from build123d import *

# Parameters (mm, degrees)
BOSS_EXTRUDE1_DEPTH      = 20.32
SKETCH2_W                = 58.42
SKETCH2_H                = 52.07
BOSS_EXTRUDE2_DEPTH      = 3.81
SKETCH3_W                = 12.7
SKETCH3_H                = 20.32
CUT_EXTRUDE1_DEPTH       = 3.81
FILLET2_R                = 2.54
SKETCH4_W                = 10.16
SKETCH4_H                = 5.08
BOSS_EXTRUDE3_DEPTH      = 10.16
CHAMFER1_SIZE            = 0.762
SKETCH5_W                = 10.16
SKETCH5_H                = 5.08
BOSS_EXTRUDE4_DEPTH      = 10.16
CHAMFER2_SIZE            = 0.762
CHAMFER2_OF_MIRROR1_SIZE = 0.762
M3_CLEARANCE_HOLE1_D     = 3.4
M3_CLEARANCE_HOLE2_D     = 3.4
CUT_EXTRUDE2_REACH       = 61.966
SKETCH13_W               = 44.45
SKETCH13_H               = 16.51
SKETCH15_W               = 13.462
SKETCH15_H               = 7.366
CUT_EXTRUDE4_DEPTH       = 79.475827011
FILLET3_R                = 2.54
SKETCH16_W               = 6.35
SKETCH16_H               = 3.81
BOSS_EXTRUDE5_DEPTH      = 3.81
CHAMFER3_SIZE            = 0.762
M3_CLEARANCE_HOLE4_D     = 3.4
CUT_EXTRUDE5_DEPTH       = 3.302


with BuildPart() as part:
    # Sketch1 → Boss-Extrude1 (new body)
    with BuildSketch(Plane(origin=(0, 0, 0), x_dir=(1, 0, 0), z_dir=(0, 1, 0))):
        Polygon((-27.305, 22.225), (-27.305, 26.035), (31.115, 26.035), (31.115, -26.035), (-27.305, -26.035), (-27.305, -22.225), (27.305, -22.225), (27.305, 22.225), align=None)
    extrude(amount=BOSS_EXTRUDE1_DEPTH)

    # Sketch2 → Boss-Extrude2 (add)
    with BuildSketch(Plane(origin=(0, 20.32, 0), x_dir=(1, 0, 0), z_dir=(0, 1, 0))):
        with Locations((1.905, 0)):
            Rectangle(SKETCH2_W, SKETCH2_H)
    extrude(amount=BOSS_EXTRUDE2_DEPTH)

    # Sketch3 → Cut-Extrude1 (cut)
    with BuildSketch(Plane.ZY.offset(-27.305)):
        with Locations((-15.875, 10.16)):
            Rectangle(SKETCH3_W, SKETCH3_H)
        with Locations((15.875, 10.16)):
            Rectangle(SKETCH3_W, SKETCH3_H)
    extrude(amount=-CUT_EXTRUDE1_DEPTH, mode=Mode.SUBTRACT)

    # Fillet2
    fillet2_edges = [part.edges().sort_by_distance(p)[0] for p in [
        (31.115, 12.065, -26.035),
        (31.115, 12.065, 26.035),
        (31.115, 24.13, 0),
    ]]
    fillet(fillet2_edges, radius=FILLET2_R)

    # Sketch4 → Boss-Extrude3 (add)
    with BuildSketch(Plane(origin=(31.115, 0, 0), x_dir=(0, 0, -1), z_dir=(1, 0, 0))):
        with Locations((0, 2.54)):
            Rectangle(SKETCH4_W, SKETCH4_H)
    extrude(amount=BOSS_EXTRUDE3_DEPTH)

    # Chamfer1
    chamfer1_edges = [part.edges().sort_by_distance(p)[0] for p in [
        (31.115, 2.54, 5.08),
        (36.195, 5.08, 5.08),
        (31.115, 2.54, -5.08),
        (31.115, 5.08, 0),
        (36.195, 5.08, -5.08),
        (41.275, 2.54, 5.08),
        (41.275, 2.54, -5.08),
        (41.275, 5.08, 0),
    ]]
    chamfer(chamfer1_edges, length=CHAMFER1_SIZE)

    # Sketch5 → Boss-Extrude4 (add)
    with BuildSketch(Plane.XY.offset(26.035)):
        with Locations((-14.605, 2.54)):
            Rectangle(SKETCH5_W, SKETCH5_H)
    boss_extrude4 = extrude(amount=BOSS_EXTRUDE4_DEPTH)

    # Chamfer2
    chamfer2_edges = [part.edges().sort_by_distance(p)[0] for p in [
        (-19.685, 2.54, 26.035),
        (-19.685, 5.08, 31.115),
        (-9.525, 2.54, 26.035),
        (-14.605, 5.08, 26.035),
        (-9.525, 5.08, 31.115),
        (-19.685, 2.54, 36.195),
        (-9.525, 2.54, 36.195),
        (-14.605, 5.08, 36.195),
    ]]
    chamfer(chamfer2_edges, length=CHAMFER2_SIZE)

    # Mirror1: Boss-Extrude4 across plane
    add(boss_extrude4.mirror(Plane.XY))

    # Chamfer2 of Mirror1
    chamfer2_of_mirror1_edges = [part.edges().sort_by_distance(p)[0] for p in [
        (-19.685, 2.54, -26.035),
        (-19.685, 5.08, -31.115),
        (-9.525, 2.54, -26.035),
        (-14.605, 5.08, -26.035),
        (-9.525, 5.08, -31.115),
        (-19.685, 2.54, -36.195),
        (-9.525, 2.54, -36.195),
        (-14.605, 5.08, -36.195),
    ]]
    chamfer(chamfer2_of_mirror1_edges, length=CHAMFER2_OF_MIRROR1_SIZE)

    # M3 Clearance Hole1 (through all)
    with Locations(Plane(origin=(0, 5.08, 0), x_dir=(1, 0, 0), z_dir=(0, 1, 0))):
        with Locations((-14.605, -31.115)):
            m3_clearance_hole1 = Hole(M3_CLEARANCE_HOLE1_D / 2)

    # Mirror2: M3 Clearance Hole1 across plane
    add(m3_clearance_hole1.mirror(Plane.XY), mode=Mode.SUBTRACT)

    # M3 Clearance Hole2 (through all)
    with Locations(Plane(origin=(0, 5.08, 0), x_dir=(1, 0, 0), z_dir=(0, 1, 0))):
        with Locations((36.195, 0)):
            Hole(M3_CLEARANCE_HOLE2_D / 2)

    # Sketch13 → Cut-Extrude2 (cut, up to next)
    with BuildSketch(Plane(origin=(0, 24.13, 0), x_dir=(1, 0, 0), z_dir=(0, 1, 0)), mode=Mode.PRIVATE) as cut_extrude2_sk1:
        with Locations((0, -10.795)):
            Rectangle(SKETCH13_W, SKETCH13_H)
    cut_extrude2_tool1 = extrude(cut_extrude2_sk1.sketch, amount=-CUT_EXTRUDE2_REACH, mode=Mode.PRIVATE) & part.part
    # Sketch13 → Cut-Extrude2 (cut, up to next)
    with BuildSketch(Plane(origin=(0, 24.13, 0), x_dir=(1, 0, 0), z_dir=(0, 1, 0)), mode=Mode.PRIVATE) as cut_extrude2_sk2:
        with Locations((0, 10.795)):
            Rectangle(SKETCH13_W, SKETCH13_H)
    cut_extrude2_tool2 = extrude(cut_extrude2_sk2.sketch, amount=-CUT_EXTRUDE2_REACH, mode=Mode.PRIVATE) & part.part
    add(cut_extrude2_tool1.solids().sort_by_distance((0, 24.13, 10.795))[0], mode=Mode.SUBTRACT)
    add(cut_extrude2_tool2.solids().sort_by_distance((0, 24.13, -10.795))[0], mode=Mode.SUBTRACT)

    # Sketch15 → Cut-Extrude4 (cut, through all)
    with BuildSketch(Plane(origin=(0, 0, -26.035), x_dir=(-1, 0, 0), z_dir=(0, 0, -1))):
        Polygon((-22.225, 0), (4.953, 0), (4.953, 9.652), (4.953, 17.018), (2.441043817, 17.018), (-22.225, 17.018), align=None)
        with Locations((15.494, 13.335)):
            Rectangle(SKETCH15_W, SKETCH15_H)
    extrude(amount=-CUT_EXTRUDE4_DEPTH, mode=Mode.SUBTRACT)

    # Fillet3
    fillet3_edges = [part.edges().sort_by_distance(p)[0] for p in [
        (-22.225, 22.225, 19.05),
        (-22.225, 22.225, 2.54),
        (1.905, 20.32, -22.225),
        (22.225, 22.225, 2.54),
        (22.225, 22.225, 19.05),
        (22.225, 22.225, -19.05),
        (22.225, 22.225, -2.54),
        (-22.225, 22.225, -2.54),
        (-22.225, 22.225, -19.05),
        (22.225, 17.018, 24.13),
        (22.225, 17.018, -24.13),
        (-4.953, 17.018, 24.13),
        (-4.953, 17.018, -24.13),
        (-22.225, 17.018, 24.13),
        (-22.225, 17.018, -24.13),
        (-22.225, 9.652, 24.13),
        (-22.225, 9.652, -24.13),
        (-8.763, 9.652, 24.13),
        (-8.763, 9.652, -24.13),
        (-8.763, 17.018, 24.13),
        (-8.763, 17.018, -24.13),
        (29.21, 20.32, -9.525),
        (29.21, 20.32, 9.525),
        (1.905, 20.32, 22.225),
    ]]
    fillet(fillet3_edges, radius=FILLET3_R)

    # Sketch16 → Boss-Extrude5 (add)
    with BuildSketch(Plane(origin=(0, 24.13, 0), x_dir=(1, 0, 0), z_dir=(0, 1, 0))):
        with Locations((-27.305, 0)):
            Rectangle(SKETCH16_W, SKETCH16_H)
    extrude(amount=-BOSS_EXTRUDE5_DEPTH)

    # Chamfer3
    chamfer3_edges = [part.edges().sort_by_distance(p)[0] for p in [
        (-28.8925, 20.32, -1.905),
        (-28.8925, 20.32, 1.905),
        (-30.48, 20.32, 0),
        (-30.48, 22.225, -1.905),
        (-30.48, 22.225, 1.905),
    ]]
    chamfer(chamfer3_edges, length=CHAMFER3_SIZE)

    # M3 Clearance Hole4 (through all)
    with Locations(Plane(origin=(0, 24.13, 0), x_dir=(1, 0, 0), z_dir=(0, 1, 0))):
        with Locations((25.286866606, -21.9964), (25.286866606, 21.9964)):
            Hole(M3_CLEARANCE_HOLE4_D / 2)

    # Sketch22 → Cut-Extrude5 (cut)
    with BuildSketch(Plane.XZ.offset(-20.32)):
        Polygon((28.953040816, 21.9964), (27.119953711, 25.1714), (23.453779502, 25.1714), (21.620692397, 21.9964), (23.453779502, 18.8214), (27.119953711, 18.8214), align=None)
        Polygon((28.953040816, -21.9964), (27.119953711, -18.8214), (23.453779502, -18.8214), (21.620692397, -21.9964), (23.453779502, -25.1714), (27.119953711, -25.1714), align=None)
    extrude(amount=CUT_EXTRUDE5_DEPTH, mode=Mode.SUBTRACT)


solid = part.part
The listing builds one solid part. Answer for the finished solid, in the listing's coordinates (mm). A direction names the side the tool comes from. Round coordinates to 2 decimals unless told otherwise and drop trailing zeros. Write each loop counter-clockwise with the first axis right and the second up, starting at its lowest first coordinate (ties: lowest second). Pieces come first, ordered by that corner, then holes. Notation, with made-up numbers: M -23,39.25 L 17,39.25 A22 cw 17,61.25 Z; hole C -25.75,-20 d9. An arc over 180 degrees is marked long. Write each question's results on one line, items separated by ' | '. Start each with the question number.
Item 1: For faces 1 (the face through (28.05, 18.69, 23.56)), 2 (the face through (38.1, 5.08, 0.1)), 3 (the face through (29.237, 19.596, -10.289)), 4 (the face through (-21.461, 10.376, 24.157)), determine the directions among +Z, -Z, +X, -X, +Y, -Y from which every point of the face is accessible in a straight line to the end or side of a thin tool.
Item 2: Straight lines are drawn through the part: L1, parallel to Z at x = -10.5, y = 21.5 (3 decimals); L2, parallel to Z at x = -16, y = 2 (3 decimals); L3, parallel to Y at x = -26.5, z = 5. For each, find the intervals that lie inside material, in ascending order. Write a range as [from, to].
Item 3: A cutting plane is placed at D-D on y = 2.5. State how many separate pieces and enclosed holes the cut face has, and give its area (3 significant figures).
Item 4: A cutting plane is placed at A-A on x = -7.5. Write down the section's boundary in (y, z) (3 decimals).
Item 5: Flat-ended cylindrical pins translate along their axes: pin 1 Ø1.3 at (y, z) = (2.5, 31) entering from -X (3 decimals); pin 2 Ø4 at (x, y) = (-3, 9) entering from +Z (3 decimals); pin 3 Ø1.2 at (x, y) = (-29, 23) entering from +Z (3 decimals). Find the tip coordinate at first contact, or state that the pin passes through.
Item 6: A cutting plane is placed at B-B on y = 8. Write down the section's boundary in (x, z) (3 decimals).
Item 7: A cutting plane is placed at C-C on z = 0. Write down the section's boundary in (x, y) (3 decimals), and give its area (3 significant figures).
Item 8: For a pull along X with two mould halves and no side action, classify faces 5 (the face through (25.253, 8.39, -23.696)), 6 (the face through (30.35, 12.23, 25.31)), 7 (the face through (33, 0, 0)) as pulls with the +X half, pulls with the -X half, needs draft (parallel to the pull), parting line crosses it, or undercut.
Check sheet entries:
1) face 1: none | face 2: +Z, -Z, +X, +Y | face 3: +X, -X, -Y | face 4: +Z, -Z
2) L1: [-26.035, -19.05], [-2.54, 2.54], [19.05, 26.035] | L2: [-36.195, -32.087], [-30.143, -22.225], [22.225, 30.143], [32.087, 36.195] | L3: [20.32, 24.13]
3) separate pieces: 5 | enclosed holes: 3 | area: 583 mm²
4) outline: M 0,-26.035 L 24.13,-26.035 L 24.13,-19.05 L 20.32,-19.05 L 20.32,-19.685 A2.54 cw 17.78,-22.225 L 0,-22.225 Z; M 0,22.225 L 17.78,22.225 A2.54 cw 20.32,19.685 L 20.32,19.05 L 24.13,19.05 L 24.13,26.035 L 0,26.035 Z; M 20.32,-2.54 L 24.13,-2.54 L 24.13,2.54 L 20.32,2.54 Z
5) pin 1: x = -19.685 | pin 2: z = 26.035 | pin 3: z = 1.905
6) outline: M -27.305,-26.035 L -4.953,-26.035 L -4.953,-22.225 L -27.305,-22.225 Z; M -27.305,22.225 L -4.953,22.225 L -4.953,26.035 L -27.305,26.035 Z; M 22.225,-26.035 L 28.575,-26.035 A2.54 ccw 31.115,-23.495 L 31.115,-22.225 L 26.971,-22.225 A1.7 cw 23.602,-22.225 L 22.225,-22.225 Z; M 22.225,22.225 L 23.602,22.225 A1.7 cw 26.971,22.225 L 31.115,22.225 L 31.115,23.495 A2.54 ccw 28.575,26.035 L 22.225,26.035 Z; M 27.305,-9.525 L 31.115,-9.525 L 31.115,9.525 L 27.305,9.525 Z
7) outline: M -30.48,21.082 L -29.718,20.32 L 27.305,20.32 L 27.305,0 L 34.495,0 L 34.495,5.08 L 31.877,5.08 L 31.115,5.842 L 31.115,21.59 A2.54 ccw 28.575,24.13 L -30.48,24.13 Z; M 37.895,0 L 41.275,0 L 41.275,4.318 L 40.513,5.08 L 37.895,5.08 Z | area: 345 mm²
8) face 5: undercut | face 6: pulls with the +X half | face 7: needs draft
